Source: CAD feature listing. Evaluate the final solid. Frame: model axes, mm. Face numbers are marked on the shaded views. A direction names the side the tool comes from. Give positions to 0.01 mm unless a question says otherwise; leave off trailing zeros. Order: outer loops, then holes, each group sorted by start corner. A loop starts at its lowest first (then second) coordinate and runs counter-clockwise, first axis right, second up.
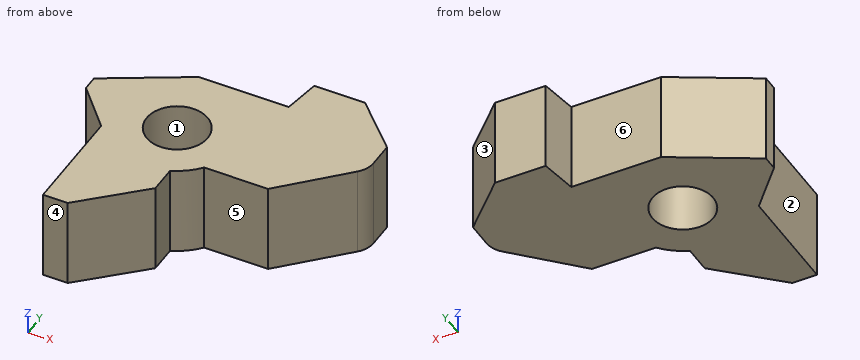
from build123d import *

# Parameters (mm, degrees)
SKETCH_1_R      = 2.515
EXTRUDE_1_DEPTH = 7.5
FILLET_1_R      = 2


with BuildPart() as part:
    # 스케치1 → 보스-돌출1 (new body)
    with BuildSketch(Plane.XY):
        with BuildLine():
            Line((-8.053143001, 0.978578295), (-5, -2.40902013))
            Line((-5, -2.40902013), (-5, -11.436332264))
            Line((-5, -11.436332264), (-2.956819065, -11.436332264))
            Line((-2.956819065, -11.436332264), (1.87605446, -6.923867857))
            Line((1.87605446, -6.923867857), (1.87605446, -4.634697365))
            ThreePointArc((1.87605446, -4.634697365), (2.980195691, -4.014776911), (3.893195608, -3.13736003))
            Line((3.893195608, -3.13736003), (9.172978659, -3.13736003))
            Line((9.172978659, -3.13736003), (14.557074242, 2.286312605))
            Line((14.557074242, 2.286312605), (14.557074242, 5.198022376))
            Line((14.557074242, 5.198022376), (10.725649804, 9.001488547))
            Line((10.725649804, 9.001488547), (6.528593017, 9.001488547))
            Line((6.528593017, 9.001488547), (6.037882178, 5.957406269))
            Line((6.037882178, 5.957406269), (-1.376355668, 5.957406269))
            Line((-1.376355668, 5.957406269), (-8.053143001, 2.219229384))
            Line((-8.053143001, 2.219229384), (-8.053143001, 0.978578295))
        make_face()
        Circle(SKETCH_1_R, mode=Mode.SUBTRACT)
    extrude(amount=EXTRUDE_1_DEPTH)

    # 필렛1
    fillet_1_edges = [part.edges().sort_by_distance(p)[0] for p in [
        (14.557074242, 2.286312605, 3.75),
    ]]
    fillet(fillet_1_edges, radius=FILLET_1_R)


solid = part.part
1) Section query C-C on x = 11.5. Output: boundary loops of the cut face in (y, z).
Checks:
outline: (-0.79, 0) - (8.23, 0) - (8.23, 7.5) - (-0.79, 7.5) - close
2) Ray query, L1, parallel to X at y = -6.5, z = 7; L2, parallel to Y at x = 0, z = 4 (3 decimals); L3, parallel to Y at x = 1, z = 3. Return the intervals inside material, ascending.
Checks:
L1: x = -5 to 1.88
L2: y = -8.676 to -2.515, 2.515 to 5.957
L3: y = -7.74 to -2.31, 2.31 to 5.96
3) Section query B-B on x = 0. Output: boundary loops of the cut face in (y, z) (3 decimals).
Checks:
outline: (-8.676, 0) - (-2.515, 0) - (-2.515, 7.5) - (-8.676, 7.5) - close; (2.515, 0) - (5.957, 0) - (5.957, 7.5) - (2.515, 7.5) - close
4) Pull-direction query (Y, two-part tool) for the marked faces 1, 2 and 3; classes: +Y half, -Y half, draft (parallel to the pull), parting line (faces both ways), or undercut.
Checks:
face 1: undercut
face 2: draft
face 3: +Y half
5) Section query A-A on z = 3.25. Output: boundary loops of the cut face in (x, y) (3 decimals), and give its area (3 significant figures).
Checks:
outline: (-8.053, 0.979) - (-5, -2.409) - (-5, -11.436) - (-2.957, -11.436) - (1.876, -6.924) - (1.876, -4.635) arc R5 ccw to (3.893, -3.137) - (9.173, -3.137) - (13.976, 1.701) arc R2 ccw to (14.557, 3.11) - (14.557, 5.198) - (10.726, 9.001) - (6.529, 9.001) - (6.038, 5.957) - (-1.376, 5.957) - (-8.053, 2.219) - close; hole circle Ø5.03 at (0, 0)
area: 217 mm2
6) First-contact query: pin 1 Ø3 at (x, z) = (-5, 1.5) entering from +Y; pin 2 Ø1 at (x, z) = (-2.5, 4.5) entering from +Y; pin 3 Ø0.7 at (y, z) = (-6, 3) entering from +X; pin 4 Ø4 at (x, y) = (9.5, -5.5) entering from -Z. Flat tips, straight axial feed; report the tip coordinate or a pass-through.
Checks:
pin 1: stops at y = 4.77
pin 2: stops at y = 5.61
pin 3: stops at x = 1.88
pin 4: passes through
7) Reachability of the marked faces 4, 5 and 6 from +Z, -Z, +X, -X, +Y, -Y: full face, straight path, thin tool, end or side. Return the list, or none.
Checks:
face 4: +Z, -Z, +X, -X, -Y
face 5: +Z, -Z, +X, -Y
face 6: +Z, -Z, -X, +Y
